Drawing for the job (mm, zero at the part's lowest x, y, z). Round coordinates to 2 decimals unless told otherwise and drop trailing zeros. Loops run counter-clockwise (first coordinate to the right, second up) from the corner with the lowest first, then second, coordinate; pieces in that order, holes last. Notation, with made-up numbers: M 77,49.25 L 104,49.25 A30 cw 104,87.25 Z; hole C 13.25,77 d3. An arc over 180 degrees is marked long. Answer in a Markdown table with one row per item.
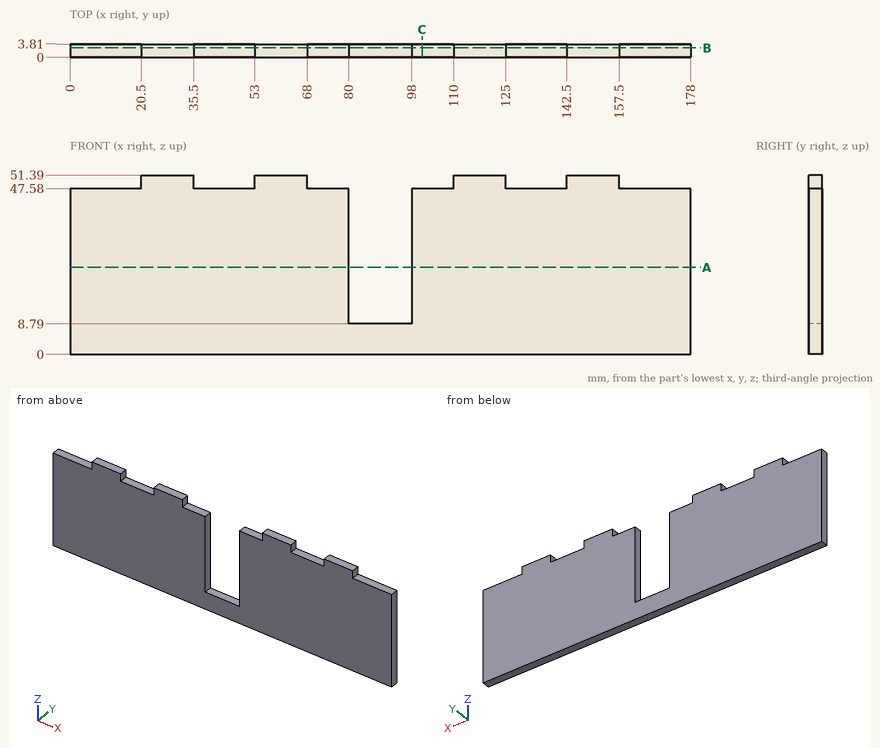
1. Saw through at B-B (y = 2.7). Write the cut outline in (x, z), and give its area (3 significant figures).
Verdict:
| item | result |
|---|---|
| outline | M 0,0 L 178,0 L 178,47.58 L 157.5,47.58 L 157.5,51.39 L 142.5,51.39 L 142.5,47.58 L 125,47.58 L 125,51.39 L 110,51.39 L 110,47.58 L 98,47.58 L 98,8.79 L 80,8.79 L 80,47.58 L 68,47.58 L 68,51.39 L 53,51.39 L 53,47.58 L 35.5,47.58 L 35.5,51.39 L 20.5,51.39 L 20.5,47.58 L 0,47.58 Z |
| area | 8,000 mm² |
2. Pin check, flat tips, straight feed: pin 1 (1.1 mm diameter, centred on y = 2.5, z = 49, fed in from -X); pin 2 (12 mm diameter, centred on x = 86.5, z = 42, fed in from -Y) (3 decimals); pin 3 (1 mm diameter, centred on x = 75, y = 1.5, fed in from +Z); pin 4 (1.9 mm diameter, centred on y = 2.5, z = 50.5, fed in from +X). Stop position of each tip, or through.
Verdict:
| item | result |
|---|---|
| pin 1 | stops at x = 20.5 |
| pin 2 | passes through |
| pin 3 | stops at z = 47.58 |
| pin 4 | stops at x = 157.5 |
3. Wall check: probe 1 along X at (y, z) = (3.4, 48); probe 2 along X at (y, z) = (1.7, 29); probe 3 along Z at (x, y) = (11.5, 2.25). Give the ranges that are in metal, low to high.
Verdict:
| item | result |
|---|---|
| probe 1 | x = 20.5 to 35.5, 53 to 68, 110 to 125, 142.5 to 157.5 |
| probe 2 | x = 0 to 80, 98 to 178 |
| probe 3 | z = 0 to 47.58 |
4. Saw through at C-C (x = 101). Write the cut outline in (y, z), and give its area (3 significant figures).
Verdict:
| item | result |
|---|---|
| outline | M 0,0 L 3.81,0 L 3.81,47.58 L 0,47.58 Z |
| area | 181 mm² |
5. Saw through at A-A (z = 25). Write the cut outline in (x, y).
Verdict:
| item | result |
|---|---|
| outline | M 0,0 L 80,0 L 80,3.81 L 0,3.81 Z; M 98,0 L 178,0 L 178,3.81 L 98,3.81 Z |
